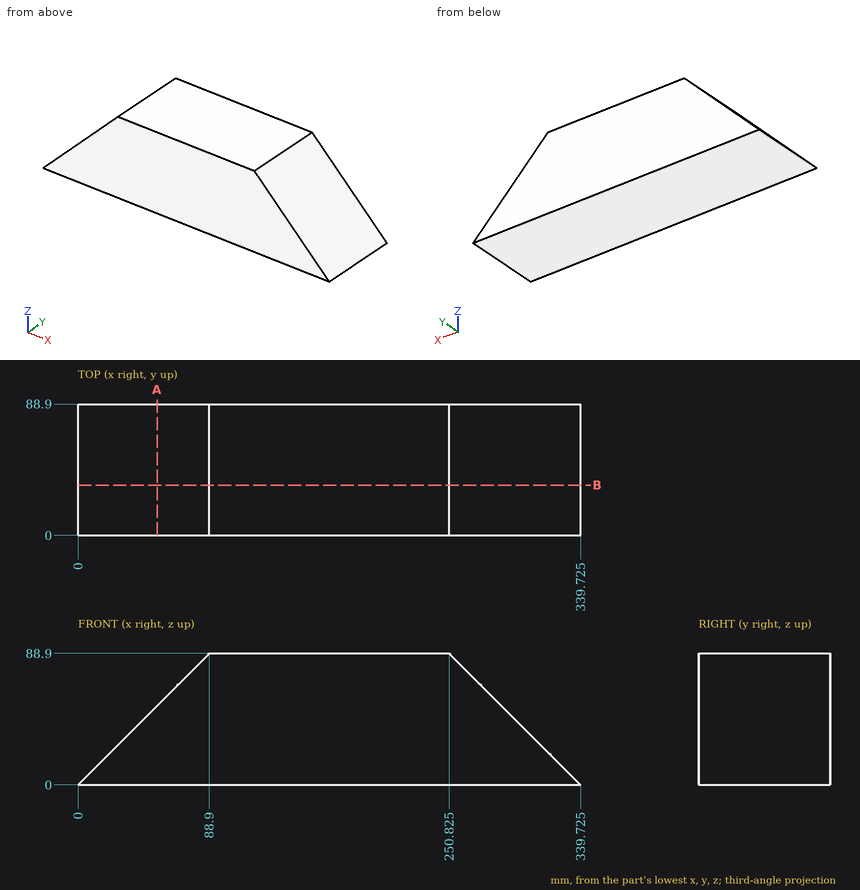
Geometry: see drawing. Coordinates: mm, zero at the bounding-box minimum. Coordinates: 2 decimals unless noted, no trailing zeros. Write each loop counter-clockwise with the first axis right and the second up, starting at its lowest first coordinate (ties: lowest second). Pieces come first, ordered by that corner, then holes. Notation, with made-up numbers: M -24.5,6 L 7.5,6 A23 ccw 7.5,40 Z; hole C -8,54.5 d11. An arc over 180 degrees is marked long. Use CSV: the item, a comma, the result in double quotes. Start each with the question number.
1. First-contact query: P1, Ø3, axis at y = 32, z = 80, coming from the -X side; P2, Ø6, axis at y = 70.5, z = 49.5, coming from the +X side (3 decimals); P3, Ø3, axis at x = 291.5, y = 51.5, coming from the +Z side (3 decimals). Flat tips, straight axial feed; report the tip coordinate or a pass-through.
2. Cut plane B-B on y = 34. Return the cut outline in (x, z) (3 decimals).
3. Ray query, probe 1 along X at (y, z) = (57, 12) (3 decimals); probe 2 along Z at (x, y) = (39, 37); probe 3 along X at (y, z) = (38.5, 65) (3 decimals). Return the intervals inside material, ascending.
4. Cut plane A-A on x = 53.5. Return the cut outline in (y, z).
Entries:
1,P1,"x = 78.5"
1,P2,"x = 293.225"
1,P3,"z = 49.725"
2,outline,"M 0,0 L 339.725,0 L 250.825,88.9 L 88.9,88.9 Z"
3,probe 1,"12 to 327.725"
3,probe 2,"0 to 39"
3,probe 3,"65 to 274.725"
4,outline,"M 0,0 L 88.9,0 L 88.9,53.5 L 0,53.5 Z"
